```python
from build123d import *

# Parameters (mm, degrees)
F0_W     = 187.772378
F0_H     = 73.266328
F1_DEPTH = 25.4
F2_R     = 5.08
F3_W     = 13.028179
F3_H     = 12.178514
F4_DEPTH = 25.4


with BuildPart() as f1:
    # F0 (on Front) → F1 (new body, symmetric)
    with BuildSketch(Plane.XZ):
        Rectangle(F0_W, F0_H)
    extrude(amount=F1_DEPTH, both=True)

    # F2
    f2_edges = [f1.edges().sort_by_distance(p)[0] for p in [
        (93.886189, -25.4, 0),
        (93.886189, 25.4, 0),
        (-93.886189, -25.4, 0),
        (-93.886189, 25.4, 0),
    ]]
    fillet(f2_edges, radius=F2_R)

    # F3 (on face) → F4 (join)
    with BuildSketch(Plane(origin=(0, 0, -36.633164), x_dir=(1, 0, 0), z_dir=(0, 0, -1))):
        with Locations((-23.224139, 0)):
            Rectangle(F3_W, F3_H)
    extrude(amount=F4_DEPTH)


solid = f1.part
```
For this review, take the finished solid that the model builds, in its own axes (mm). A direction names the side the tool comes from. Round coordinates to 2 decimals unless told otherwise and drop trailing zeros. Write each loop counter-clockwise with the first axis right and the second up, starting at its lowest first coordinate (ties: lowest second). Pieces come first, ordered by that corner, then holes. Notation, with made-up numbers: (-16.75, 88) - (41.25, 88) arc R21 ccw to (41.25, 122) - close; hole circle Ø9 at (3.5, 22). An arc over 180 degrees is marked (long way). Write each question's results on one line, items separated by ' | '.
Item 1: To check wall thickness, follow line 1 along Z through (x, y) = (80.5, -15.5); line 2 along X through (y, z) = (23, -16.5); line 3 along X through (y, z) = (22, 19). State the ranges of each line that lie inside material, in increasing order. Write a range as from..to.
Calculated:
line 1: z = -36.63..36.63 | line 2: x = -93.12..93.12 | line 3: x = -93.6..93.6
Item 2: Take a section at B-B on z = -42. State the section outline as (x, y) points, then the cut area to 3 significant figures.
Calculated:
outline: (-29.74, -6.09) - (-16.71, -6.09) - (-16.71, 6.09) - (-29.74, 6.09) - close | area: 159 mm^2
Item 3: Take a section at A-A on y = 4. State the section outline as (x, z) points, then the cut area to 3 significant figures.
Calculated:
outline: (-93.89, -36.63) - (-29.74, -36.63) - (-29.74, -62.03) - (-16.71, -62.03) - (-16.71, -36.63) - (93.89, -36.63) - (93.89, 36.63) - (-93.89, 36.63) - close | area: 14,100 mm^2
Item 4: For faces 1 (the face through (-23, -6.089, -49)), 2 (the face through (-23, 6.089, -49)), 3 (the face through (-29.738, 0, -49)), list the 3-axis set-ups (+Z, -Z, +X, -X, +Y, -Y) from which the entire face can be reached by the end or side of a thin tool; tool diameter is ignored.
Calculated:
face 1: -Z, +X, -X, -Y | face 2: -Z, +X, -X, +Y | face 3: -Z, -X, +Y, -Y
Item 5: For pin 1 (13.5 mm diameter, centred on y = -1, z = -48, fed in from -X); pin 2 (6.5 mm diameter, centred on x = -26.5, z = -54.5, fed in from -Y); pin 3 (13.5 mm diameter, centred on y = -3, z = -45, fed in from +X), all flat-tipped, find the tip position at first contact; note any pin that passes through.
Calculated:
pin 1: stops at x = -29.74 | pin 2: stops at y = -6.09 | pin 3: stops at x = -16.71
Item 6: Take a section at C-C on x = -61.5. State the section outline as (y, z) points.
Calculated:
outline: (-25.4, -36.63) - (25.4, -36.63) - (25.4, 36.63) - (-25.4, 36.63) - close
